Input: dimensioned drawing with shaded views. Units: mm. Origin: part minimum x, y, z. A direction names the side the tool comes from. Give positions to 0.01 mm unless a question says otherwise; leave off trailing zeros. Write each loop counter-clockwise with the first axis right and the second up, starting at its lowest first coordinate (ties: lowest second). Pieces come first, ordered by that corner, then holes.
Q1. Line query: line 1 (Z direction, x = 3, y = 39.5); line 2 (Y direction, x = 3, z = 30); line 3 (X direction, y = 62, z = 213). Output: solid intervals per line, ascending.
Q2. Section C-C (x = 36). Return the cut outline in (y, z), plus the area to 3 significant figures.
Q3. Section A-A (z = 30). Return the cut outline in (x, y).
Q4. Section B-B (y = 35). Return the cut outline in (x, z).
Q5. Reachability of the marked faces 1 and 2 from +Z, -Z, +X, -X, +Y, -Y: full face, straight path, thin tool, end or side. Return the list, or none.
Q6. Pin query (flat end, axial travel): pin 1 Ø6 at (x, y) = (10, 52.5) entering from -Z; pin 2 Ø1.5 at (x, z) = (41.5, 50.5) entering from -Y; pin 3 Ø12 at (x, z) = (30.5, 93.5) entering from +Y; pin 4 Ø24 at (y, z) = (35, 30) entering from +X. Return the tip coordinate at first contact, or that it passes through.
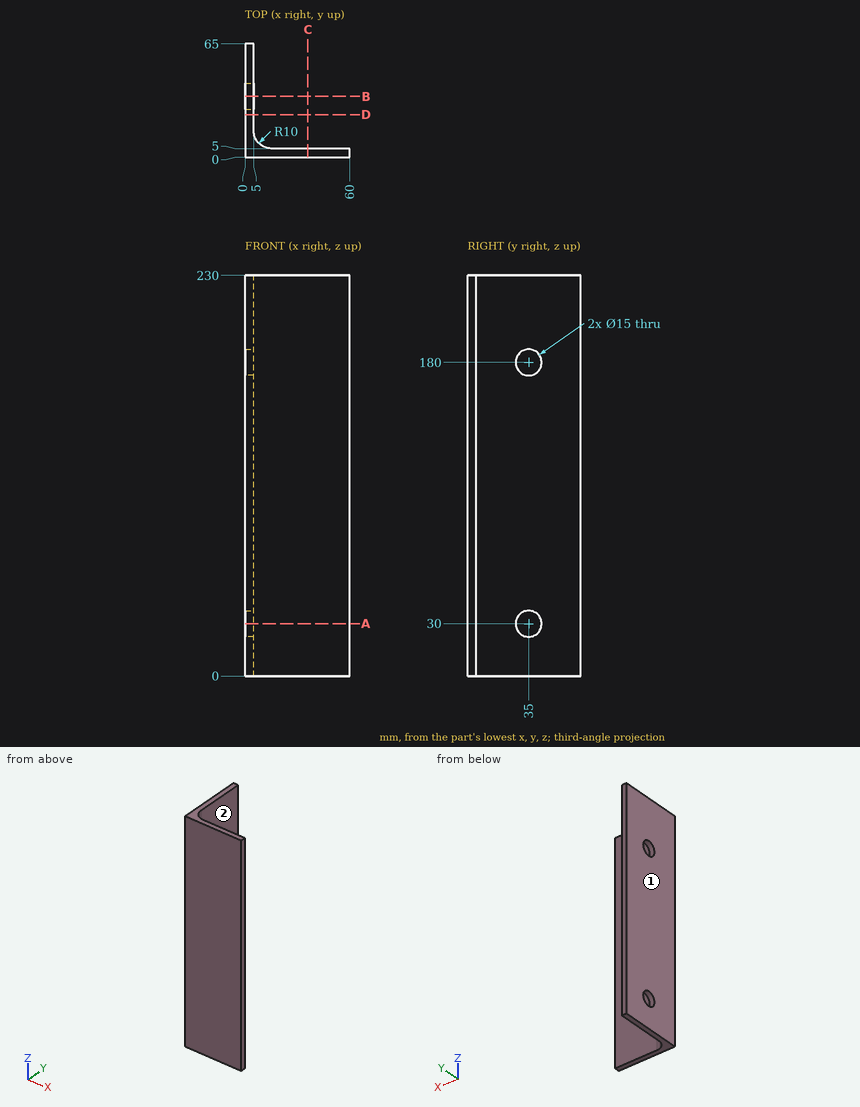
Computed:
1. line 1: z = 0 to 24, 36 to 174, 186 to 230
1. line 2: y = 0 to 27.5, 42.5 to 65
1. line 3: x = 0 to 5
2. outline: (0, 0) - (5, 0) - (5, 230) - (0, 230) - close
2. area: 1,150 mm2
3. outline: (0, 0) - (60, 0) - (60, 5) - (15, 5) arc R10 cw to (5, 15) - (5, 27.5) - (0, 27.5) - close; (0, 42.5) - (5, 42.5) - (5, 65) - (0, 65) - close
4. outline: (0, 0) - (5, 0) - (5, 22.5) - (0, 22.5) - close; (0, 37.5) - (5, 37.5) - (5, 172.5) - (0, 172.5) - close; (0, 187.5) - (5, 187.5) - (5, 230) - (0, 230) - close
5. face 1: +Z, -Z, -X, +Y, -Y
5. face 2: +Z, -Z, +X, +Y
6. pin 1: passes through
6. pin 2: stops at y = 0
6. pin 3: stops at y = 5
6. pin 4: stops at x = 5
